Check sheet for the modelled part. Datum: model origin and axes. Units: mm. A direction names the side the tool comes from. Give positions to 0.01 mm unless a question says otherwise; leave off trailing zeros. Order: outer loops, then holes, each group sorted by start corner. A loop starts at its lowest first (then second) coordinate and runs counter-clockwise, first axis right, second up. Notation, with made-up numbers: (39.5, -1) -> (85.5, -1) arc R35 ccw to (85.5, 33) -> close; hole circle Ø10 at (3, 86). An arc over 180 degrees is marked (long way). One line per question, with ' | ' between items.
```python
from build123d import *

# Parameters (mm, degrees)
F0_W        = 5
F0_H        = 5
F0_W_2      = 40
F0_H_2      = 238
F1_DEPTH    = 80
F2_T4_DEPTH = 80
F2_T7_DEPTH = 328.751226723


# Not quite as in the source:
# - a fillet or chamfer that OpenCascade refuses, or shapes differently, is made with other operations: its cross-section is extruded or revolved along the edge and cut away or added


with BuildPart() as f1:
    # F0 (on Top) → F1 (new body)
    with BuildSketch(Plane.XY):
        with Locations((0, -119)):
            Rectangle(F0_W, F0_H)
        with Locations((-22.5, -119)):
            Rectangle(F0_W_2, F0_H)
        with Locations((0, 2.5)):
            Rectangle(F0_W, F0_H_2)
    extrude(amount=F1_DEPTH)

    # F2: fillet of radius 50 on 2 edges, made by hand


with BuildPart() as f2_tool2:
    # F2_s3 → F2_t4 (new body)
    with BuildSketch(Plane.XY):
        with BuildLine():
            ThreePointArc((-2.4996, -67.5094166718), (-13.7698250279, -99.1327516284), (-42.4999199938, -116.5003919171))
            Line((-42.4999199938, -116.5003919171), (-41.4998154247, -121.3994894416))
            ThreePointArc((-41.4998154247, -121.3994894416), (-22.4999599969, -121.5001365685), (-2.5, -121.5001365685))
            Line((-2.5, -121.5001365685), (2.5001365685, -116.5))
            ThreePointArc((2.5001365685, -116.5), (2.5001365685, -92.0047083359), (2.5005365685, -67.5094166718))
            Line((2.5005365685, -67.5094166718), (-2.4996, -67.5094166718))
        make_face()
    extrude(amount=F2_T4_DEPTH)

    split(bisect_by=Plane.YZ.offset(2.5), keep=Keep.BOTTOM)

    split(bisect_by=Plane.XZ.offset(121.5), keep=Keep.BOTTOM)


with BuildPart() as f1_1:
    add(f1.part)

    # F2_t1: union F2_tool2
    add(f2_tool2.part)

    # F2_s8 → F2_t7 (cut)
    with BuildSketch(Plane.XY.offset(-124.3756133615)):
        with BuildLine():
            ThreePointArc((2.5004, -71.749754657), (-10.4186674501, -105.2913665442), (-42.499959993, -121.5003979943))
            Line((-42.499959993, -121.5003979943), (-41.9998594238, -126.475462328))
            ThreePointArc((-41.9998594238, -126.475462328), (-19.9999799965, -126.5001365685), (2.5, -126.5001365685))
            Line((2.5, -126.5001365685), (7.5001365685, -121.5))
            ThreePointArc((7.5001365685, -121.5), (7.5001365685, -96.6248773285), (7.5005365685, -71.749754657))
            Line((7.5005365685, -71.749754657), (2.5004, -71.749754657))
        make_face()
    extrude(amount=F2_T7_DEPTH, mode=Mode.SUBTRACT)


solid = f1_1.part
```
Q1. Section check B-B (y = -42). Enter the section's corners in (x, z), and give its area (3 significant figures).
Result sheet:
outline: (-2.5, 0) -> (2.5, 0) -> (2.5, 80) -> (-2.5, 80) -> close | area: 400 mm2
Q2. Access from +Z, -Z, +X, -X, +Y, -Y to the whole of each face (thin tool, end or side, straight path). Record for faces 1 (the face through (-2.5, 26, 39)), 2 (the face through (-10.14, -104.98, 39.44)).
Result sheet:
face 1: +Z, -Z, -X, +Y | face 2: +Z, -Z, +X, -Y
Q3. Section check C-C (x = -14). Enter the section's corners in (y, z), and give its area (3 significant figures).
Result sheet:
outline: (-108.87, 0) -> (-99.41, 0) -> (-99.41, 80) -> (-108.87, 80) -> close | area: 756 mm2
Q4. Thickness scan on line 1 (X direction, y = 102, z = 34); line 2 (Y direction, x = -32, z = 41.5); line 3 (Y direction, x = -11, z = 67). Record the ranges inside material, lowest first.
Result sheet:
line 1: x = -2.5 to 2.5 | line 2: y = -119.29 to -113.11 | line 3: y = -105.92 to -95.4
Q5. Depth check by flat-ended pin: pin 1 Ø5 at (y, z) = (-26.5, 56) entering from -X; pin 2 Ø2 at (x, z) = (-21, 46.5) entering from -Y; pin 3 Ø10 at (x, z) = (-15.5, 68.5) entering from -Y. Enter the tip coordinate at first touch or a pass-through.
Result sheet:
pin 1: stops at x = -2.5 | pin 2: stops at y = -114.76 | pin 3: stops at y = -113.83
